The drawing under review shows one solid part. Ordinate dimensions are in mm from its lowest x, y, z. A direction names the side the tool comes from. Give positions to 0.01 mm unless a question says otherwise; leave off trailing zeros. Write each loop counter-clockwise with the first axis right and the second up, starting at its lowest first coordinate (ties: lowest second). Pieces come first, ordered by that corner, then holes. Notation, with made-up numbers: M -3.5,-17 L 28.5,-17 A27 cw 28.5,10 Z; hole C 64,1 d4. An arc over 180 degrees is marked long. Write item = value, one per line. Start each with the question number.
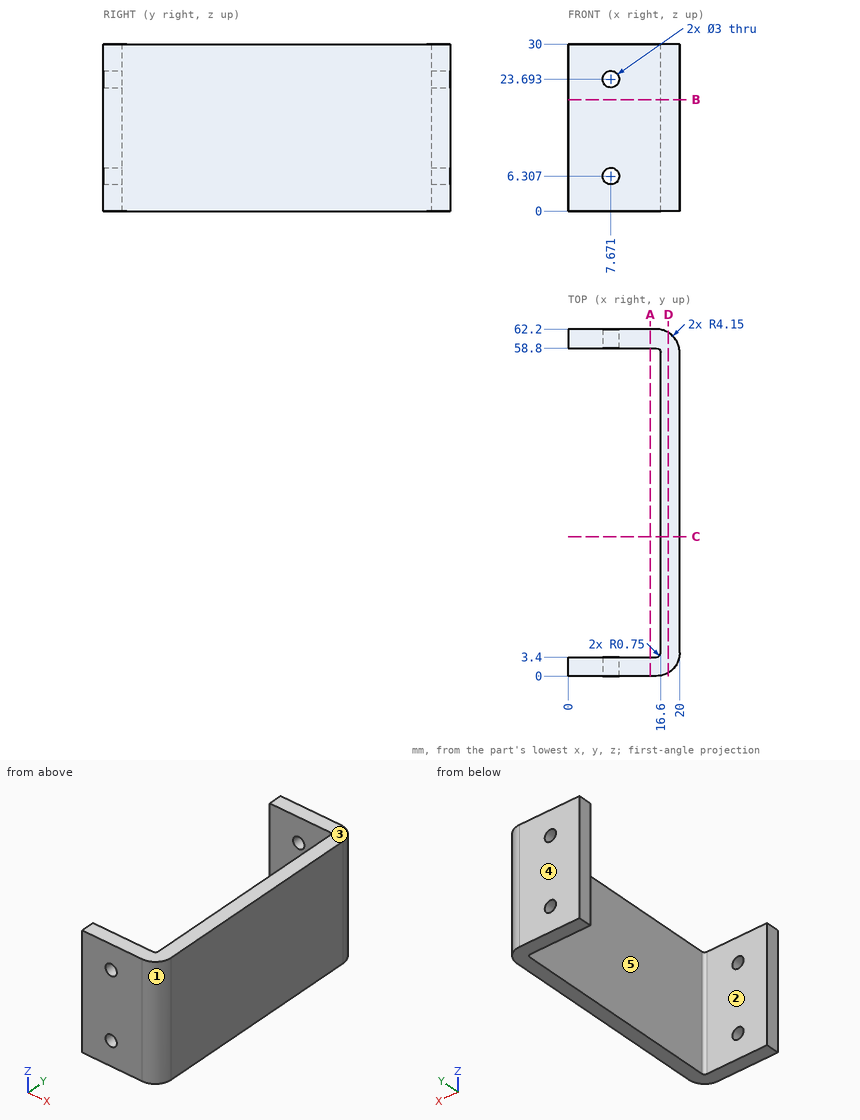
Item 1: We need section C-C, the plane y = 25. Write out the cut boundary in (x, z).
Item 2: Clearance check with flat-ended pins moving along their axes: P1, Ø1.8, axis at x = 7.67, z = 6.31, coming from the -Y side; P2, Ø1.5, axis at y = 6.5, z = 17, coming from the -X side; P3, Ø5, axis at x = 7.67, z = 6.31, coming from the -Y side. State where each tip first meets the part, or that it passes through.
Item 3: We need section D-D, the plane x = 18. Write out the cut boundary in (y, z), and give its area (3 significant figures).
Item 4: We need section A-A, the plane x = 14.75. Write out the cut boundary in (y, z), and give its area (3 significant figures).
Item 5: For the marked faces 1 and 2, list the 3-axis set-ups (+Z, -Z, +X, -X, +Y, -Y) from which the entire face can be reached by the end or side of a thin tool; tool diameter is ignored.
Item 6: To check wall thickness, follow probe 1 along Y at (x, z) = (11.25, 5.25); probe 2 along X at (y, z) = (42, 15.25); probe 3 along Y at (x, z) = (17.25, 10.75). State the ranges of each line that lie inside material, in increasing order. Write a range as [from, to].
Item 7: We need section B-B, the plane z = 20. Write out the cut boundary in (x, y), and give its area (3 significant figures).
Item 8: The part is to be moulded in two halves that separate along Y. For the marked faces 3, 4 and 5, say which applies: released by +Y, released by -Y, zero draft, split by the parting line, or undercut.
Worked out:
q1.outline = M 16.6,0 L 20,0 L 20,30 L 16.6,30 Z
q2.P1 = through
q2.P2 = 16.6
q2.P3 = 0
q3.outline = M 0.6,0 L 61.6,0 L 61.6,30 L 0.6,30 Z
q3.area = 1,830 mm²
q4.outline = M 0,0 L 3.4,0 L 3.4,30 L 0,30 Z; M 58.8,0 L 62.2,0 L 62.2,30 L 58.8,30 Z
q4.area = 204 mm²
q5.face_1 = +Z, -Z, +X, -Y
q5.face_2 = +Z, -Z, -X
q6.probe_1 = [0, 3.4], [58.8, 62.2]
q6.probe_2 = [16.6, 20]
q6.probe_3 = [0.24, 61.96]
q7.outline = M 0,0 L 15.85,0 A4.15 ccw 20,4.15 L 20,58.05 A4.15 ccw 15.85,62.2 L 0,62.2 L 0,58.8 L 15.85,58.8 A0.75 cw 16.6,58.05 L 16.6,4.15 A0.75 cw 15.85,3.4 L 0,3.4 Z
q7.area = 317 mm²
q8.face_3 = zero draft
q8.face_4 = released by +Y
q8.face_5 = undercut
